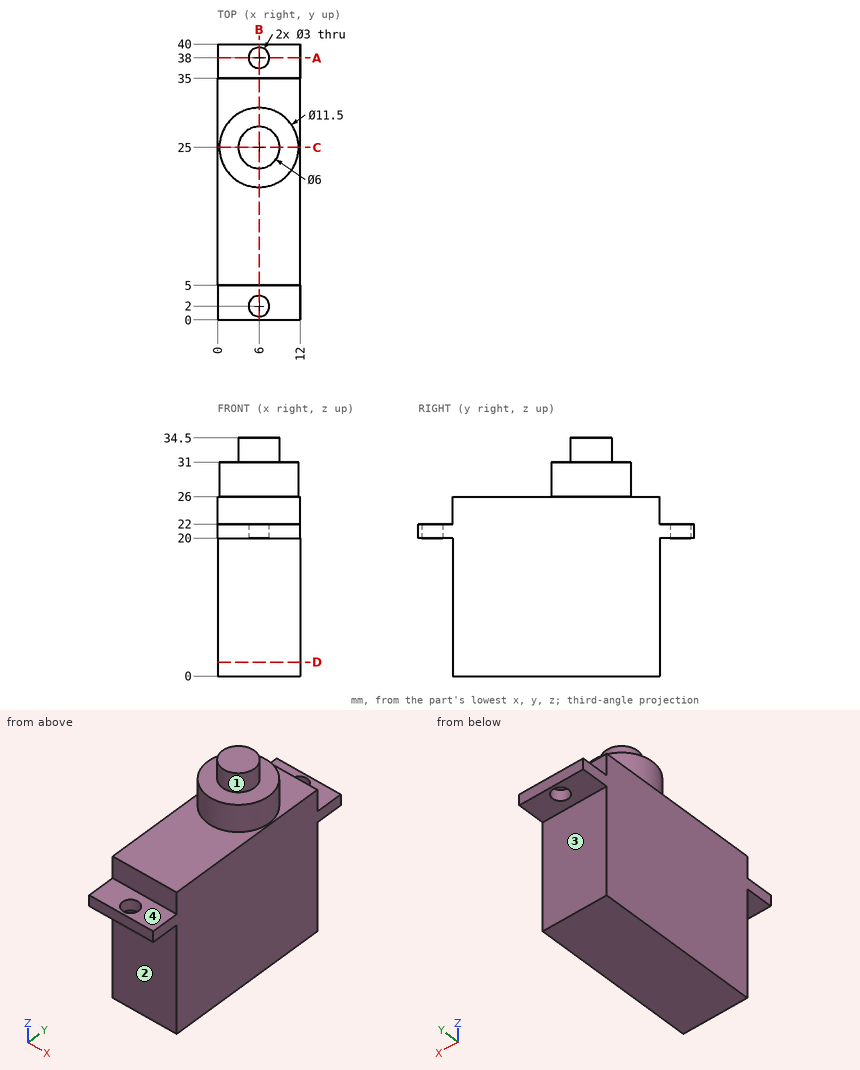
Check sheet for the drawn part. Datum: minimum x, y, z corner. Units: mm. A direction names the side the tool comes from. Give positions to 0.01 mm unless a question says otherwise; leave off trailing zeros. Order: outer loops, then holes, each group sorted by start corner. A loop starts at its lowest first (then second) coordinate and runs counter-clockwise, first axis right, second up. Notation, with made-up numbers: (65.25, 82) -> (100.25, 82) arc R14 cw to (100.25, 89) -> close; hole circle Ø6 at (9, 88.25). An arc over 180 degrees is marked (long way). Use a Markdown table: item, result.
1) Tool access check on the marked faces 1, 2, 3 and 4. Record the directions out of +Z, -Z, +X, -X, +Y, -Y that give a thin tool (end or side, any length) a straight path to the whole face; none if there is none.
Results:
| item | result |
|---|---|
| face 1 | +Z |
| face 2 | -Z, +X, -X, -Y |
| face 3 | -Z, +X, -X, +Y |
| face 4 | +Z, +X, -X, -Y |
2) Section check A-A, the plane y = 38. Record the boundary of the cut face in (x, z).
Results:
| item | result |
|---|---|
| outline | (0, 20) -> (4.5, 20) -> (4.5, 22) -> (0, 22) -> close; (7.5, 20) -> (12, 20) -> (12, 22) -> (7.5, 22) -> close |
3) Material ranges on probe 1 along Y at (x, z) = (6, 21.1); probe 2 along Z at (x, y) = (1.5, 21.5); probe 3 along Z at (x, y) = (9.25, 18), recorded low to high.
Results:
| item | result |
|---|---|
| probe 1 | 0 to 0.5, 3.5 to 36.5, 39.5 to 40 |
| probe 2 | 0 to 31 |
| probe 3 | 0 to 26 |
4) Depth check by flat-ended pin: pin 1 Ø1.5 at (x, y) = (6, 3) entering from +Z; pin 2 Ø3 at (y, z) = (30.5, 26) entering from -X; pin 3 Ø2.5 at (x, y) = (4.5, 2) entering from -Z; pin 4 Ø6 at (x, z) = (5.5, 9) entering from -Y. Enter the tip coordinate at first touch or a pass-through.
Results:
| item | result |
|---|---|
| pin 1 | z = 22 |
| pin 2 | x = 0 |
| pin 3 | z = 20 |
| pin 4 | y = 5 |
5) Section check D-D, the plane z = 2. Record the boundary of the cut face in (x, y), then the cut area to 3 significant figures.
Results:
| item | result |
|---|---|
| outline | (0, 5) -> (12, 5) -> (12, 35) -> (0, 35) -> close |
| area | 360 mm² |
6) Section check C-C, the plane y = 25. Record the boundary of the cut face in (x, z), then the cut area to 4 significant figures.
Results:
| item | result |
|---|---|
| outline | (0, 0) -> (12, 0) -> (12, 26) -> (11.75, 26) -> (11.75, 31) -> (9, 31) -> (9, 34.5) -> (3, 34.5) -> (3, 31) -> (0.25, 31) -> (0.25, 26) -> (0, 26) -> close |
| area | 390.5 mm² |
7) Section check B-B, the plane x = 6. Record the boundary of the cut face in (y, z).
Results:
| item | result |
|---|---|
| outline | (0, 20) -> (0.5, 20) -> (0.5, 22) -> (0, 22) -> close; (3.5, 20) -> (5, 20) -> (5, 0) -> (35, 0) -> (35, 20) -> (36.5, 20) -> (36.5, 22) -> (35, 22) -> (35, 26) -> (30.75, 26) -> (30.75, 31) -> (28, 31) -> (28, 34.5) -> (22, 34.5) -> (22, 31) -> (19.25, 31) -> (19.25, 26) -> (5, 26) -> (5, 22) -> (3.5, 22) -> close; (39.5, 20) -> (40, 20) -> (40, 22) -> (39.5, 22) -> close |
